Here's the drawing with two shaded views (mm, measured from the low corner). I have some questions. Coordinates: 2 decimals unless noted, no trailing zeros. Write each loop counter-clockwise with the first axis right and the second up, starting at its lowest first coordinate (ties: lowest second). Pieces come first, ordered by that corner, then holes. Notation, with made-up numbers: M 34.5,76.25 L 41.5,76.25 A23 ccw 41.5,109.25 Z; hole C -16.75,-7 d8. An arc over 180 degrees is marked long. Answer as CSV lines item,"result". Start each with the question number.
Item 1: If I drill on line 1 along Y through (x, z) = (2.3, 15); line 2 along Y through (x, z) = (5, 78.5); line 3 along Z through (x, y) = (3, 138.5), over which ranges is the centre line in solid material (lowest first)? Write a range as [from, to].
Item 2: I'm going to push flat-ended pins straight in: P1, Ø1.5, axis at y = 106, z = 40.5, coming from the -X side; P2, Ø3, axis at x = 1.5, z = 72.5, coming from the +Y side; P3, Ø3, axis at y = 77, z = 83.5, coming from the +X side; P4, Ø1.5, axis at x = 2.5, y = 122, coming from the +Z side. Where does each tip first touch, or does it pass through?
Item 3: Suppose I cut it at C-C, the plane x = 1.1. Write out the boundary of the cut face in (y, z).
Item 4: Suppose I cut it at B-B, the plane z = 15. Write out the boundary of the cut face in (x, y), and give its area (3 significant figures).
Item 5: Suppose I cut it at D-D, the plane z = 77. Write out the boundary of the cut face in (x, y).
Item 6: Suppose I cut it at A-A, the plane y = 135. Write out the boundary of the cut face in (x, z), and give its area (3 significant figures).
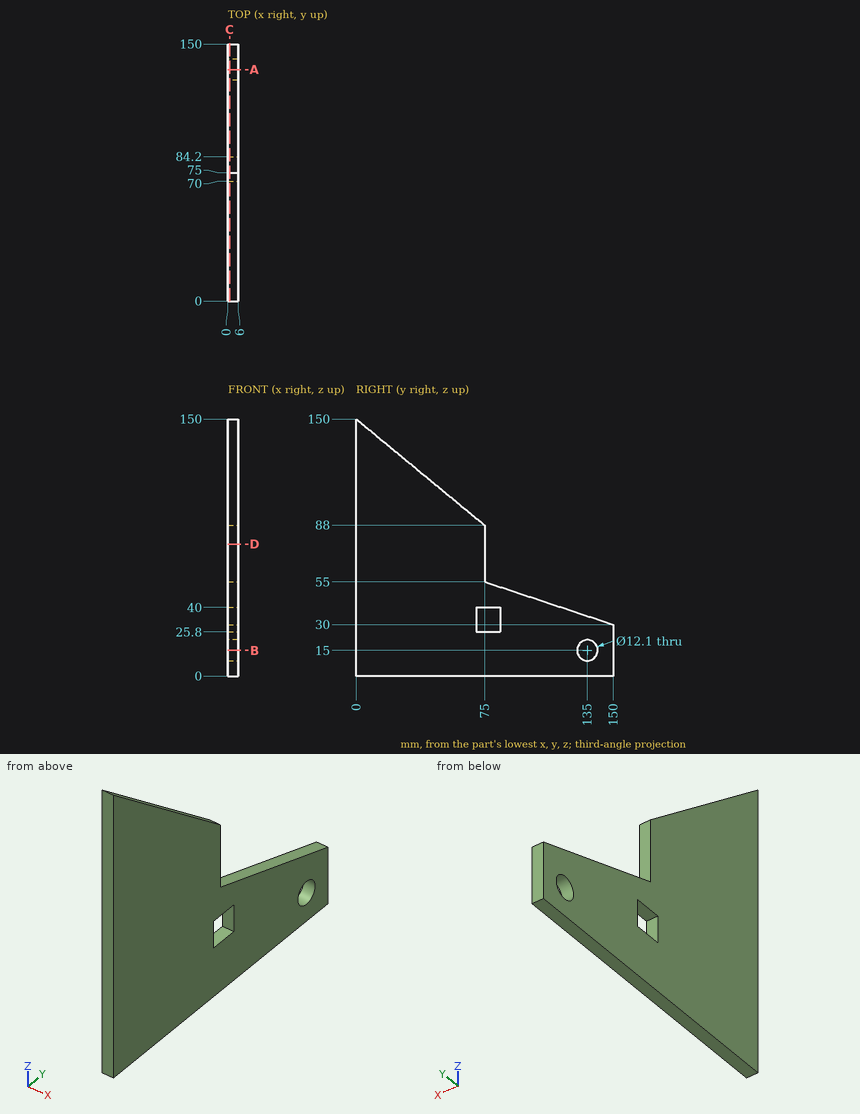
Ans:
1,line 1,"y = [0, 128.95], [141.05, 150]"
1,line 2,"y = [0, 75]"
1,line 3,"z = [0, 10.07], [19.93, 33.83]"
2,P1,"stops at x = 0"
2,P2,"stops at y = 75"
2,P3,"passes through"
2,P4,"stops at z = 39.58"
3,outline,"M 0,0 L 150,0 L 150,30 L 75,55 L 75,88 L 0,150 Z; hole M 70,25.8 L 84.2,25.8 L 84.2,40 L 70,40 Z; hole C 135,15 d12.1"
4,outline,"M 0,0 L 6,0 L 6,128.95 L 0,128.95 Z; M 0,141.05 L 6,141.05 L 6,150 L 0,150 Z"
4,area,"827 mm^2"
5,outline,"M 0,0 L 6,0 L 6,75 L 0,75 Z"
6,outline,"M 0,0 L 6,0 L 6,8.95 L 0,8.95 Z; M 0,21.05 L 6,21.05 L 6,35 L 0,35 Z"
6,area,"137 mm^2"
